Geometry: final body of the model. Coordinates: model frame, mm. A direction names the side the tool comes from. Coordinates: 2 decimals unless noted, no trailing zeros. Write each loop counter-clockwise with the first axis right and the second up, starting at its lowest first coordinate (ties: lowest second). Pieces come first, ordered by that corner, then holes. Notation, with made-up numbers: (13, 31) -> (17, 31) arc R24 ccw to (17, 66) -> close; hole circle Ø5 at (7.5, 20). An arc over 180 degrees is marked (long way). One line per item, written item: value. Start each with the question number.
from build123d import *

# Parameters (mm, degrees)
MOTOR_HOLDER_DEPTH  = 12
SKETCH2_R           = 1.7
BOSS_EXTRUDE1_DEPTH = 3
FILLET1_R           = 5


with BuildPart() as part:
    # Sketch1 → Motor Holder (new body)
    with BuildSketch(Plane(origin=(0, 0, 0), x_dir=(0, 0, -1), z_dir=(1, 0, 0))):
        with BuildLine():
            Line((-8.387700817, 10.61), (8.387700817, 10.61))
            ThreePointArc((8.387700817, 10.61), (13.525, 0), (8.387700817, -10.61))
            Line((8.387700817, -10.61), (-8.387700817, -10.61))
            ThreePointArc((-8.387700817, -10.61), (-13.525, 0), (-8.387700817, 10.61))
        make_face()
        with BuildLine():
            Line((-7.923037612, 9.31), (7.923037612, 9.31))
            ThreePointArc((7.923037612, 9.31), (12.225, 0), (7.923037612, -9.31))
            Line((7.923037612, -9.31), (-7.923037612, -9.31))
            ThreePointArc((-7.923037612, -9.31), (-12.225, 0), (-7.923037612, 9.31))
        make_face(mode=Mode.SUBTRACT)
    extrude(amount=MOTOR_HOLDER_DEPTH)

    # Sketch2 → Boss-Extrude1 (add)
    # profile 1 of 4: a face of its own
    with BuildSketch(Plane.ZY):
        with BuildLine():
            Line((-15.86201317, 5.433547478), (-12.795120435, 4.382980497))
            ThreePointArc((-12.795120435, 4.382980497), (-11.039561677, 7.8136869), (-8.387700817, 10.61))
            Line((-8.387700817, 10.61), (-15, 10.61))
            ThreePointArc((-15, 10.61), (-17.623867728, 8.386941811), (-15.86201317, 5.433547478))
        make_face()
        with Locations((-15, 7.95)):
            Circle(SKETCH2_R, mode=Mode.SUBTRACT)
    # profile 2 of 4: a face of its own
    with BuildSketch(Plane.ZY):
        with BuildLine():
            Line((-15, -10.61), (-8.387700817, -10.61))
            ThreePointArc((-8.387700817, -10.61), (-11.039561677, -7.8136869), (-12.795120435, -4.382980497))
            Line((-12.795120435, -4.382980497), (-15.86201317, -5.433547478))
            ThreePointArc((-15.86201317, -5.433547478), (-17.623867728, -8.386941811), (-15, -10.61))
        make_face()
        with Locations((-15, -7.95)):
            Circle(SKETCH2_R, mode=Mode.SUBTRACT)
    # profile 3 of 4: a face of its own
    with BuildSketch(Plane.ZY):
        with BuildLine():
            Line((15.86201317, -5.433547478), (12.795120435, -4.382980497))
            ThreePointArc((12.795120435, -4.382980497), (11.039561677, -7.8136869), (8.387700817, -10.61))
            Line((8.387700817, -10.61), (15, -10.61))
            ThreePointArc((15, -10.61), (17.623867728, -8.386941811), (15.86201317, -5.433547478))
        make_face()
        with Locations((15, -7.95)):
            Circle(SKETCH2_R, mode=Mode.SUBTRACT)
    # profile 4 of 4: a face of its own
    with BuildSketch(Plane.ZY):
        with BuildLine():
            Line((15, 10.61), (8.387700817, 10.61))
            ThreePointArc((8.387700817, 10.61), (11.039561677, 7.8136869), (12.795120435, 4.382980497))
            Line((12.795120435, 4.382980497), (15.86201317, 5.433547478))
            ThreePointArc((15.86201317, 5.433547478), (17.623867728, 8.386941811), (15, 10.61))
        make_face()
        with Locations((15, 7.95)):
            Circle(SKETCH2_R, mode=Mode.SUBTRACT)
    extrude(amount=-BOSS_EXTRUDE1_DEPTH)

    # Fillet1
    # the kernel refuses this fillet: 5 mm, written as the material it adds along each edge
    with BuildSketch(Plane(origin=(0, -4.382980497, -12.795120435), x_dir=(0, -0.3311587269792296, -0.9435750619561202), z_dir=(1, 0, 0)), Plane(origin=(0, 4.382980497, 12.795120435), x_dir=(0, 0.3311587269792292, 0.9435750619561204), z_dir=(1, 0, 0))) as fillet1_piece_1:
        with BuildLine():
            CenterArc((4.297165601, 4.954108155), FILLET1_R, 195.837486713, 66.393727894)
            Line((-0.513032618, 3.589559476), (-0.99405244, 3.453104608))
            ThreePointArc((-0.99405244, 3.453104608), (-0.630646565, 1.74130771), (-0.499985908, -0.003753963))
            Line((-0.499985908, -0.003753963), (0.003753963, -0.499985908))
            ThreePointArc((0.003753963, -0.499985908), (3.245501889, -0.475646418), (3.553698727, -0.495410815))
            Line((3.553698727, -0.495410815), (3.621286625, 0))
        make_face()
    extrude(amount=3)
    with BuildSketch(Plane(origin=(0, 4.382980497, -12.795120435), x_dir=(0, 0.3311587269792287, -0.9435750619561205), z_dir=(1, 0, 0)), Plane(origin=(0, -4.382980497, 12.795120435), x_dir=(0, -0.3311587269792296, 0.9435750619561202), z_dir=(1, 0, 0))) as fillet1_piece_2:
        with BuildLine():
            CenterArc((4.297165601, -4.954108155), FILLET1_R, 97.768785393, 66.393727894)
            Line((-0.513032618, -3.589559476), (-0.99405244, -3.453104608))
            ThreePointArc((-0.99405244, -3.453104608), (-0.630646565, -1.74130771), (-0.499985908, 0.003753963))
            Line((-0.499985908, 0.003753963), (0.003753963, 0.499985908))
            ThreePointArc((0.003753963, 0.499985908), (3.245501889, 0.475646418), (3.553698727, 0.495410815))
            Line((3.553698727, 0.495410815), (3.621286625, 0))
        make_face()
    extrude(amount=3)


solid = part.part
Q1. Cut plane B-B on y = 4. Output: boundary loops of the cut face in (x, z).
Q2. Cut plane C-C on x = 9.5. Output: boundary loops of the cut face in (y, z) (3 decimals).
Q3. Line query: L1, parallel to Y at x = 1.55, z = 15; L2, parallel to Y at x = 5.25, z = 7.5; L3, parallel to Z at x = 10.5, y = 1.5. Output: solid intervals per line, ascending. Write a range as from..to.
Q4. Cut plane D-D on z = -15.5. Output: boundary loops of the cut face in (x, y).
Q5. First-contact query: P1, Ø2, axis at x = 7, y = 7.5, coming from the +Z side; P2, Ø1.5, axis at x = 6.5, y = -6, coming from the -Z side. Flat tips, straight axial feed; report the tip coordinate or a pass-through.
Q6. Access query for faces 1 (the cylindrical face through (7.249, 0.171, -13.524)), 2 (the cylindrical face through (1.479, 3.573, 14.127)), 3 (the flat face through (3, -8, -13)), 4 (the flat face through (6, -9.31, 0)), 5 (the flat face through (3, 8, 13)). Directions: +Z, -Z, +X, -X, +Y, -Y. A direction counts if a zero-diameter tool reaches every point of the face in a straight line with its end or side. Return the directions, or none.
Q7. Cut plane A-A on z = -0.5. Output: boundary loops of the cut face in (x, y).
Solution:
1. outline: (0, -14.4) -> (3, -14.4) -> (3, -12.92) -> (12, -12.92) -> (12, -11.55) -> (0, -11.55) -> close; (0, 11.55) -> (12, 11.55) -> (12, 12.92) -> (3, 12.92) -> (3, 14.4) -> (0, 14.4) -> close
2. outline: (-10.61, -8.388) arc R13.525 ccw to (10.61, -8.388) -> (10.61, 8.388) arc R13.525 ccw to (-10.61, 8.388) -> close; hole (-9.31, -7.923) arc R12.225 ccw to (9.31, -7.923) -> (9.31, 7.923) arc R12.225 ccw to (-9.31, 7.923) -> close
3. L1: -10.61..-9.65, -6.25..-4.71, 4.71..6.25, 9.65..10.61
3. L2: -10.61..-9.31, 9.31..10.61
3. L3: -13.44..-12.13, 12.13..13.44
4. outline: (0, -10.56) -> (3, -10.56) -> (3, -9.57) -> (0, -9.57) -> close; (0, -6.33) -> (3, -6.33) -> (3, -5.14) -> (0, -5.14) -> close; (0, 5.14) -> (3, 5.14) -> (3, 6.33) -> (0, 6.33) -> close; (0, 9.57) -> (3, 9.57) -> (3, 10.56) -> (0, 10.56) -> close
5. P1: z = 11.86
5. P2: z = -12.46
6. face 1: -Z, +X
6. face 2: +Z, +X, -X
6. face 3: -Z, +X, -Y
6. face 4: +X, -X
6. face 5: +Z, +X, +Y
7. outline: (0, -10.61) -> (12, -10.61) -> (12, -9.31) -> (0, -9.31) -> close; (0, 9.31) -> (12, 9.31) -> (12, 10.61) -> (0, 10.61) -> close
